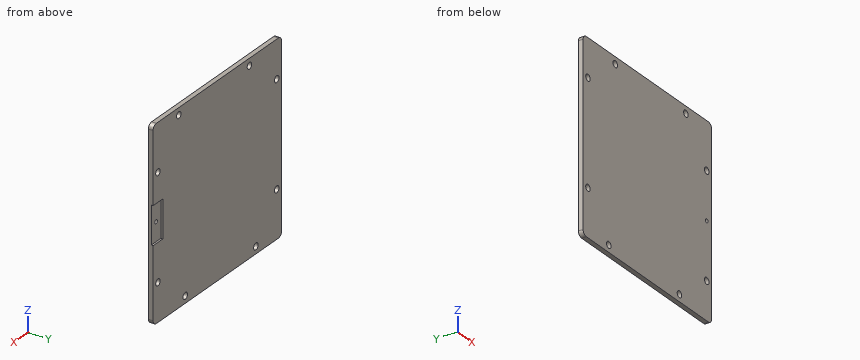
Autodesk Inventor part; units mm, degrees
ref_plane "Work Plane2" through (-195, 0, -100) normal (0, 0, 1) x (1, 0, 0)
ref_plane "YZ Plane" through (0, 0, 0) normal (1, 0, 0) x (0, 1, 0)
ref_plane "XZ Plane" through (0, 0, 0) normal (0, 1, 0) x (-1, 0, 0)
sketch "Sketch1" plane through (0, 0, 0) normal (0, 1, 0) x (-1, 0, 0)
  line L0 (0, 0) -> (200, 0)
  line L1 (200, 0) -> (200, -200)
  line L2 (200, -200) -> (0, -200)
  line L3 (0, -200) -> (0, 0)
  dimension "d0" = 200
  dimension "d1" = 200
extrude "Extrusion1" add sketch "Sketch1" along normal blind 5
fillet "Fillet2" radius 5 4 edges at (0, 2.5, 0) (0, 2.5, -200) (-200, 2.5, 0) (-200, 2.5, -200)
sketch "Sketch4" plane through (0, 5, 0) normal (0, 1, 0) x (1, 0, 0)
  circle A0 centre (-7.5, 50) radius 3.5
  circle A1 centre (-40, 7.5) radius 3.5
  line L0 (-195, 0) -> (-5, 0)
  line L1 (0, 5) -> (0, 195)
  circle A2 centre (-150, 7.5) radius 3.5
  circle A3 centre (-192.5, 40) radius 3.5
  line L2 (-200, 195) -> (-200, 5)
  circle A4 centre (-192.5, 150) radius 3.5
  circle A5 centre (-160, 192.5) radius 3.5
  circle A6 centre (-50, 192.5) radius 3.5
  circle A7 centre (-7.5, 160) radius 3.5
  line L3 (-5, 200) -> (-195, 200)
  point P0 (0, 0)
  dimension "d42" = 7
  dimension "d43" = 7
  dimension "d44" = 50
  dimension "d45" = 40
  dimension "d46" = 7.5
  dimension "d47" = 7.5
  dimension "d48" = 7
  dimension "d49" = 7
  dimension "d50" = 40
  dimension "d51" = 50
  dimension "d52" = 7.5
  dimension "d53" = 7.5
  dimension "d73" = 7.5
  dimension "d74" = 7.5
  dimension "d75" = 7.5
  dimension "d76" = 7.5
  dimension "d77" = 7
  dimension "d78" = 7
  dimension "d79" = 7
  dimension "d80" = 7
  dimension "d81" = 50
  dimension "d82" = 40
  dimension "d83" = 50
  dimension "d84" = 40
extrude "Extrusion4" cut sketch "Sketch4" against normal through all
ref_plane "Work Plane2" through (-195, 0, -100) normal (0, 0, 1) x (1, 0, 0)
sketch "Sketch5" plane through (0, 5, 0) normal (0, 1, 0) x (1, 0, 0)
  line L0 (-195, 0) -> (-5, 0)
  line L1 (-5, 200) -> (-195, 200)
  line L2 (0, 120) -> (-15, 120)
  line L3 (-15, 120) -> (-15, 80)
  line L4 (-15, 80) -> (0, 80)
  line L5 (0, 80) -> (0, 120)
  line L6 (0, 5) -> (0, 195)
  point P0 (0, 0)
  dimension "d58" = 80
  dimension "d59" = 80
  dimension "d60" = 15
  dimension "d61" = 0
extrude "Extrusion5" cut sketch "Sketch5" against normal blind 2
sketch "Sketch6" plane through (0, 3, 0) normal (0, 1, 0) x (1, 0, 0)
  line L0 (0, 120) -> (0, 80)
  line L1 (0, 80) -> (-15, 80)
  point P0 (0, 0)
  point P1 (-7.5, 100)
  dimension "d64" = 7.5
  dimension "d65" = 20
hole "Hole1" at (-7.5, 3, -100) direction (0, -1, 0) diameter 4 end through all
properties part number "top_plate"
Model file for the job. Use its own axes, mm. Coordinates: 2 decimals unless noted, no trailing zeros. Write each loop counter-clockwise with the first axis right and the second up, starting at its lowest first coordinate (ties: lowest second). Pieces come first, ordered by that corner, then holes. Notation, with made-up numbers: (35.5, 27.5) - (77.5, 27.5) arc R20 cw to (77.5, 58.5) - close; hole circle Ø6 at (50, 76). An arc over 180 degrees is marked (long way). Write each question's results on one line, items separated by ' | '. Start each with the question number.
1) Cut at A-A (z = -7.5). Write the cut outline in (x, y), then the cut area to 3 significant figures.
2) Cut at C-C (y = 3.9). Count the separate pieces of the cut face and the enclosed holes in it, then the cut area to 3 significant figures.
3) Cut at B-B (x = -150). Write the cut outline in (y, z), then the cut area to 3 significant figures.
4) Probe line 1 along X through (y, z) = (2.4, -192.5); line 2 along Z through (x, y) = (-192.5, 3.8); line 3 along Z through (x, y) = (-7.5, 2.5). List the from-to ranges inside material, lowest first. Write a range as from..to.
5) Cut at D-D (x = -192.5). Write the cut outline in (y, z), then the cut area to 3 significant figures.
6) Flat gauge pins, fed straight in: P1, Ø5.5, axis at x = -7.5, z = -50, coming from the -Y side; P2, Ø9, axis at x = -192.5, z = -150, coming from the +Y side; P3, Ø0.6, axis at y = 3.5, z = -94.5, coming from the +X side; P4, Ø4.5, axis at x = -5, z = -109, coming from the +Y side. Where does each tip first touch, or does it go through?
Returned:
1) outline: (-200, 0) - (-153.5, 0) - (-153.5, 5) - (-200, 5) - close; (-146.5, 0) - (-43.5, 0) - (-43.5, 5) - (-146.5, 5) - close; (-36.5, 0) - (0, 0) - (0, 5) - (-36.5, 5) - close | area: 930 mm^2
2) separate pieces: 1 | enclosed holes: 8 | area: 39,100 mm^2
3) outline: (0, -200) - (5, -200) - (5, -11) - (0, -11) - close; (0, -4) - (5, -4) - (5, 0) - (0, 0) - close | area: 965 mm^2
4) line 1: -200..-163.5, -156.5..-53.5, -46.5..0 | line 2: -200..-153.5, -146.5..-43.5, -36.5..0 | line 3: -200..-163.5, -156.5..-102, -98..-53.5, -46.5..0
5) outline: (0, -200) - (5, -200) - (5, -153.5) - (0, -153.5) - close; (0, -146.5) - (5, -146.5) - (5, -43.5) - (0, -43.5) - close; (0, -36.5) - (5, -36.5) - (5, 0) - (0, 0) - close | area: 930 mm^2
6) P1: through | P2: y = 5 | P3: x = -15 | P4: y = 3
